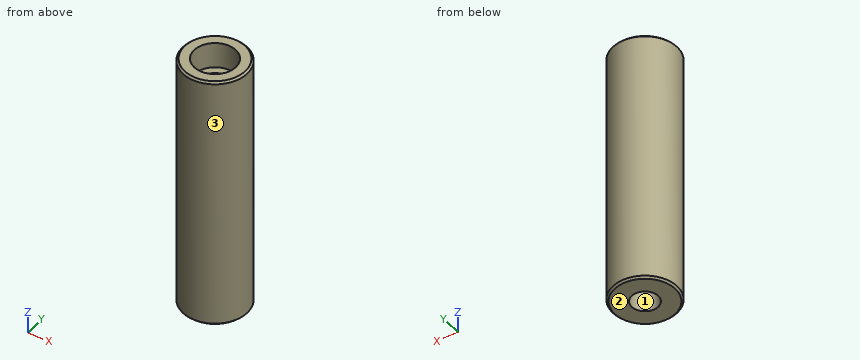
from build123d import *

# Parameters (mm, degrees)
SKETCH_1_R                = 8.5
EXTRUDE_1_DEPTH           = 68
HOLE_WIZARD_1_D           = 7
HOLE_WIZARD_1_CBORE_D     = 11
HOLE_WIZARD_1_CBORE_DEPTH = 6.8
CHAMFER_1_SIZE            = 0.5


with BuildPart() as part:
    # 草图1 → 凸台-拉伸1 (new body)
    with BuildSketch(Plane.XY):
        with Locations((-11.725470696, -50.937423366)):
            Circle(SKETCH_1_R)
    extrude(amount=EXTRUDE_1_DEPTH)

    # 打孔尺寸(%根据)内六角圆柱头螺钉的类型1 (through all)
    with Locations(Plane.XY.offset(68)):
        with Locations((-11.725470696, -50.937423366)):
            CounterBoreHole(HOLE_WIZARD_1_D / 2, HOLE_WIZARD_1_CBORE_D / 2, HOLE_WIZARD_1_CBORE_DEPTH)

    # 倒角1
    chamfer_1_edges = [part.edges().sort_by_distance(p)[0] for p in [
        (-20.225470696, -50.937423366, 0),
        (-20.225470696, -50.937423366, 68),
    ]]
    chamfer(chamfer_1_edges, length=CHAMFER_1_SIZE)


solid = part.part
Could you check a few things on this model? Use its own coordinates, in mm. Face numbers are marked on the shaded views. Coordinates: 2 decimals unless noted, no trailing zeros. Loops run counter-clockwise (first coordinate to the right, second up) from the corner with the lowest first, then second, coordinate; pieces in that order, holes last.
1. Imagine slicing it at B-B (z = 4.5). Please give me the cut outline in (x, y).
2. For P1, Ø5.5, axis at x = -9.5, y = -52, coming from the +Z side, with a flat end and sliding along its axis, tell me the tip position at first contact or that it passes through.
3. I need wall thicknesses on L1, parallel to X at y = -51.5, z = 25; L2, parallel to Z at x = -9.75, y = -56; L3, parallel to Y at x = -14.75, z = 58.5. Which ranges of each line are inside material? Lowest first, please.
4. We'd pull the mould along Y, two halves only. Please class the marked faces 1, 2 and 3: released by +Y, released by -Y, zero draft, split by the parting line, or undercut.
5. Imagine slicing it at A-A (z = 62). Please give me the cut outline in (x, y).
Computed values:
1. outline: circle Ø17 at (-11.73, -50.94); hole circle Ø7 at (-11.73, -50.94)
2. P1: stops at z = 61.2
3. L1: x = -20.21 to -15.18, -8.27 to -3.24
3. L2: z = 0 to 61.2
3. L3: y = -58.88 to -52.7, -49.18 to -42.99
4. face 1: undercut
4. face 2: zero draft
4. face 3: split by the parting line
5. outline: circle Ø17 at (-11.73, -50.94); hole circle Ø11 at (-11.73, -50.94)
